Could you check a few things on this model? Use its own coordinates, in mm. Face numbers are marked on the shaded views. A direction names the side the tool comes from. Round coordinates to 2 decimals unless told otherwise and drop trailing zeros. Order: outer loops, then holes, each group sorted by start corner. A loop starts at its lowest first (then second) coordinate and runs counter-clockwise, first axis right, second up. Notation, with made-up numbers: (28.5, 7.5) - (33.5, 7.5) arc R3 cw to (33.5, 11.5) - close; hole circle Ø11 at (-10, -5). An arc over 180 degrees is marked (long way). Use one line per item in the form item = value.
from build123d import *

# Parameters (mm, degrees)
F1_DEPTH  = 15
F2_R      = 10
F3_SIZE   = 3
F4_R      = 1
F6_DEPTH  = 25.4
F7_R      = 10
F8_DEPTH  = 1
F11_T     = -2.5
F12_W     = 7.4454136193
F12_H     = 73.2100643218
F3_FACE_W = 3.4142135624
F3_FACE_H = 81
F13_DEPTH = 81.8


# Not quite as in the source:
# - a fillet or chamfer that OpenCascade refuses, or shapes differently, is made with other operations: its cross-section is extruded or revolved along the edge and cut away or added


with BuildPart() as f1:
    # F0 (on Front) → F1 (new body)
    with BuildSketch(Plane.XZ):
        with BuildLine():
            Line((22.5, 50.5), (-22.5, 50.5))
            ThreePointArc((-22.5, 50.5), (-29.5710678119, 47.5710678119), (-32.5, 40.5))
            Line((-32.5, 40.5), (-32.5, -50.5))
            Line((-32.5, -50.5), (32.5, -50.5))
            Line((32.5, -50.5), (32.5, 40.5))
            ThreePointArc((32.5, 40.5), (29.5710678119, 47.5710678119), (22.5, 50.5))
        make_face()
    extrude(amount=F1_DEPTH)

    # F2
    f2_edges = [f1.edges().sort_by_distance(p)[0] for p in [
        (0, -15, -50.5),
    ]]
    fillet(f2_edges, radius=F2_R)

    # F3
    f3_edges = [f1.edges().sort_by_distance(p)[0] for p in [
        (32.5, -15, 0),
        (-32.5, -2.5, -50.5),
        (-32.5, -12.071068, -47.571068),
        (-32.5, -15, 0),
        (32.5, -2.5, -50.5),
        (32.5, -12.071068, -47.571068),
        (-29.571068, -15, 47.571068),
        (0, -15, 50.5),
        (29.571068, -15, 47.571068),
    ]]
    chamfer(f3_edges, length=F3_SIZE)

    # F4
    f4_edges = [f1.edges().sort_by_distance(p)[0] for p in [
        (32.5, -12, 0),
        (-32.5, -12, 0),
        (29.5, -15, 0),
        (-32.5, -2.5, -47.5),
        (-32.5, -9.949747, -45.449747),
        (-29.5, -2.5, -50.5),
        (-29.571068, -12, 47.571068),
        (-29.5, -12.071068, -47.571068),
        (-29.5, -15, 0),
        (29.5, -2.5, -50.5),
        (0, -12, 50.5),
        (32.5, -2.5, -47.5),
        (29.571068, -12, 47.571068),
        (32.5, -9.949747, -45.449747),
        (-27.449747, -15, 45.449747),
        (29.5, -12.071068, -47.571068),
        (27.449747, -15, 45.449747),
        (0, -15, 47.5),
    ]]
    fillet(f4_edges, radius=F4_R)

    # F5 (on face) → F6 (cut)
    with BuildSketch(Plane.XZ.offset(15)):
        with BuildLine():
            Line((15.5, 33.0857864376), (-15.5, 33.0857864376))
            ThreePointArc((-15.5, 33.0857864376), (-17.6213203436, 32.2071067812), (-18.5, 30.0857864376))
            Line((-18.5, 30.0857864376), (-18.5, 9.0857864376))
            ThreePointArc((-18.5, 9.0857864376), (-17.6213203436, 6.9644660941), (-15.5, 6.0857864376))
            Line((-15.5, 6.0857864376), (15.5, 6.0857864376))
            ThreePointArc((15.5, 6.0857864376), (17.6213203436, 6.9644660941), (18.5, 9.0857864376))
            Line((18.5, 9.0857864376), (18.5, 30.0857864376))
            ThreePointArc((18.5, 30.0857864376), (17.6213203436, 32.2071067812), (15.5, 33.0857864376))
        make_face()
    extrude(amount=-F6_DEPTH, mode=Mode.SUBTRACT)

    # F7 (on face) → F8 (cut)
    with BuildSketch(Plane.XZ.offset(15)):
        with Locations((0, -16.9142135624)):
            Circle(F7_R)
    extrude(amount=-F8_DEPTH, mode=Mode.SUBTRACT)

    # F9: fillet of radius 5.08 on 1 edges, made by hand

    # F9_s1 → F9_t2 (revolve)
    with BuildSketch(Plane.XY.offset(-16.9142135624)):
        with BuildLine():
            ThreePointArc((10, -15), (8.567188555, -14.2564743185), (6.9734508099, -14))
            Line((6.9734508099, -14), (10, -14))
            Line((10, -14), (10, -15))
        make_face()
    revolve(axis=Axis((0, -14, -16.9142135624), (0, -1, 0)))

    # F10: fillet of radius 4 on 1 edges, made by hand

    # F10_s1 → F10_t2 (revolve, cut)
    with BuildSketch(Plane.XY.offset(-16.9142135624)):
        with BuildLine():
            add(Edge.make_bspline(
                [(11.1159138454, -15), (10.1503047462, -15), (9.2910402615, -14.5594713656)],
                knots=[0, 0, 0, 1, 1, 1], degree=2, weights=[1, 1, 1]))
            ThreePointArc((9.2910402615, -14.5594713656), (9.6545831872, -14.7651501561), (10, -15))
            Line((10, -15), (11.1159138454, -15))
        make_face()
    revolve(axis=Axis((0, -15, -16.9142135624), (0, -1, 0)), mode=Mode.SUBTRACT)

    # F11
    f11_openings = [f1.faces().sort_by_distance(p)[0] for p in [
        (18.5, -7.5, 19.585786),
        (17.62132, -7.5, 32.207107),
        (0, -7.5, 33.085786),
        (-17.62132, -7.5, 32.207107),
        (-18.5, -7.5, 19.585786),
        (-17.62132, -7.5, 6.964466),
        (0, -7.5, 6.085786),
        (17.62132, -7.5, 6.964466),
        (0, 0, -3.809825),
    ]]
    offset(amount=F11_T, openings=f11_openings)

    # F12 (on face) + F3_face (on face) → F13 (cut)
    with BuildSketch(Plane(origin=(-32.5, 0, 0), x_dir=(0, -1, 0), z_dir=(-1, 0, 0))):
        with Locations((3.7227068096, -3.3467467874)):
            Rectangle(F12_W, F12_H)
    with BuildSketch(Plane(origin=(31, -13.5, 0), x_dir=(0.7071067812, 0.7071067812, 0), z_dir=(0.7071067812, -0.7071067812, 0))):
        Rectangle(F3_FACE_W, F3_FACE_H)
    extrude(amount=-F13_DEPTH, dir=(-1, 0, 0), mode=Mode.SUBTRACT)


solid = f1.part
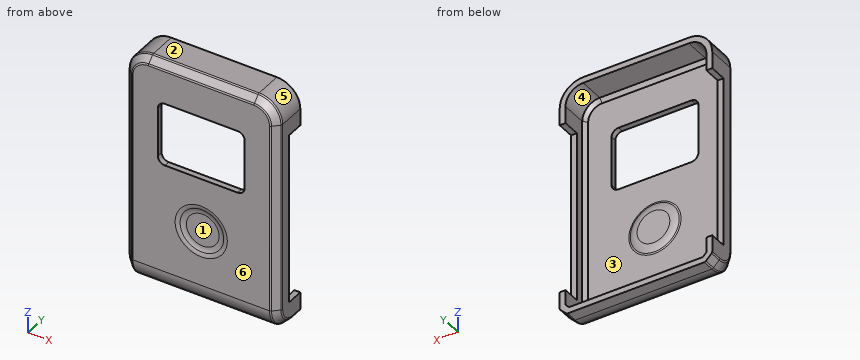
Item 1: I need wall thicknesses on L1, parallel to X at y = -8.25, z = -17; L2, parallel to Z at x = 19, y = -3.5; L3, parallel to Y at x = -10.5, z = -35. Which ranges of each line are inside material? Lowest first, please.
Found:
L1 = -32.5 to -30, 30 to 32.5
L2 = -50.5 to -48, 48 to 50.5
L3 = -15 to -12.5
Item 2: Imagine slicing it at D-D on x = 21.5. Please give me the cut outline in (y, z), plus the area to 3 significant figures.
Found:
outline = (-15, -40.5) arc R10 ccw to (-5, -50.5) - (0, -50.5) - (0, -48) - (-5, -48) arc R7.5 cw to (-12.5, -40.5) - (-12.5, 46.46) - (-10.96, 48) - (0, 48) - (0, 50.5) - (-11.59, 50.5) arc R1 ccw to (-12.29, 50.21) - (-14.71, 47.79) arc R1 ccw to (-15, 47.09) - close
area = 302 mm2
Item 3: Imagine slicing it at C-C on y = -3.25. Please give me the cut outline in (x, z).
Found:
outline = (-32.5, -47.09) arc R1 ccw to (-32.21, -47.79) - (-29.79, -50.21) arc R1 ccw to (-29.09, -50.5) - (29.09, -50.5) arc R1 ccw to (29.79, -50.21) - (32.21, -47.79) arc R1 ccw to (32.5, -47.09) - (32.5, -39.95) - (30, -39.95) - (30, -46.46) - (28.46, -48) - (-28.46, -48) - (-30, -46.46) - (-30, -39.95) - (-32.5, -39.95) - close; (-32.5, 33.26) - (-30, 33.26) - (-30, 40.5) arc R7.5 cw to (-22.5, 48) - (22.5, 48) arc R7.5 cw to (30, 40.5) - (30, 33.26) - (32.5, 33.26) - (32.5, 40.5) arc R10 ccw to (22.5, 50.5) - (-22.5, 50.5) arc R10 ccw to (-32.5, 40.5) - close
Item 4: Imagine slicing it at B-B on x = -12.5. Please give me the cut outline in (y, z).
Found:
outline = (-15, -40.5) arc R10 ccw to (-5, -50.5) - (0, -50.5) - (0, -48) - (-5, -48) arc R7.5 cw to (-12.5, -40.5) - (-12.5, 6.09) - (-15, 6.09) - close; (-15, 33.09) - (-12.5, 33.09) - (-12.5, 46.46) - (-10.96, 48) - (0, 48) - (0, 50.5) - (-11.59, 50.5) arc R1 ccw to (-12.29, 50.21) - (-14.71, 47.79) arc R1 ccw to (-15, 47.09) - close
Item 5: For the marked faces 1, 2 and 3, which set-ups out of +Z, -Z, +X, -X, +Y, -Y let a thin tool reach every point of the face, with its end or its side?
Found:
face_1 = -Y
face_2 = +Z, +X, -X, +Y, -Y
face_3 = +Y
Item 6: Imagine slicing it at A-A on z = 28. Please give me the cut outline in (x, y), plus the area to 3 significant figures.
Found:
outline = (-32.5, -11.59) arc R1 ccw to (-32.21, -12.29) - (-29.79, -14.71) arc R1 ccw to (-29.09, -15) - (-18.5, -15) - (-18.5, -12.5) - (-28.46, -12.5) - (-30, -10.96) - (-30, -7.45) - (-32.5, -7.45) - close; (18.5, -15) - (29.09, -15) arc R1 ccw to (29.79, -14.71) - (32.21, -12.29) arc R1 ccw to (32.5, -11.59) - (32.5, -7.45) - (30, -7.45) - (30, -10.96) - (28.46, -12.5) - (18.5, -12.5) - close
area = 88.5 mm2
Item 7: Will these pins go through, and if not, where does the flat tip stop? P1, Ø3.5, axis at x = 4.5, y = -7, coming from the -Z side; P2, Ø1.2, axis at x = -31.5, y = -2.5, coming from the +Z side; P3, Ø0.8, axis at x = -2.5, y = -13.5, coming from the +Z side; P4, Ø4, axis at x = -5.5, z = 9.5, coming from the +Y side.
Found:
P1 = -50.5
P2 = 45.93
P3 = 49.4
P4 = through
Item 8: If we mould it in two halves opening along X, with no side actions, what happens to the marked faces 4, 5 and 6? For each: released by +X, released by -X, zero draft, split by the parting line, or undercut.
Found:
face_4 = undercut
face_5 = released by +X
face_6 = zero draft
